from build123d import *

# Parameters (mm, degrees)
F1_DEPTH = 3.175
F2_R     = 1.984375
F3_DEPTH = 3.176


with BuildPart() as f1:
    # F0 (on Top) → F1 (new body)
    with BuildSketch(Plane.XY):
        with BuildLine():
            Line((75.480408, 88.9), (-75.480408, 88.9))
            Line((-75.480408, 88.9), (-75.480408, -88.9))
            Line((-75.480408, -88.9), (-100.880408, -88.9))
            Line((-100.880408, -88.9), (-100.880408, -101.6))
            ThreePointArc((-100.880408, -101.6), (0, -144.660291), (100.880408, -101.6))
            Line((100.880408, -101.6), (100.880408, -88.9))
            Line((100.880408, -88.9), (75.480408, -88.9))
            Line((75.480408, -88.9), (75.480408, 88.9))
        make_face()
    extrude(amount=F1_DEPTH)

    # F2 (on Top) → F3 (cut, through all)
    with BuildSketch(Plane.XY):
        with Locations((69.130408, -45.22089)):
            Circle(F2_R)
        with Locations((69.130408, -18.27911)):
            Circle(F2_R)
        with Locations((-69.130408, -45.22089)):
            Circle(F2_R)
        with Locations((-69.130408, -18.27911)):
            Circle(F2_R)
    extrude(amount=F3_DEPTH, mode=Mode.SUBTRACT)


solid = f1.part
Geometry check sheet. Reference: the model listing, model coordinates, mm. Round coordinates to 2 decimals unless told otherwise and drop trailing zeros. Order: outer loops, then holes, each group sorted by start corner. A loop starts at its lowest first (then second) coordinate and runs counter-clockwise, first axis right, second up. Notation, with made-up numbers: (12, -11) - (61, -11) arc R19 ccw to (61, 9) - close; hole circle Ø1 at (65, -25.5). An arc over 180 degrees is marked (long way). One line per question, with ' | ' between items. Start each with the question number.
(1) Sectioned sample at B-B on z = 1.1. Record the cut outline in (x, y), and give its area (3 significant figures).
(2) Depth check by flat-ended pin: pin 1 Ø2.5 at (x, y) = (69.13, -18.28) entering from +Z; pin 2 Ø1 at (y, z) = (-14.5, 1.5) entering from -X. Enter the tip coordinate at first touch or a pass-through.
(3) Sectioned sample at C-C on x = 32. Record the cut outline in (y, z) (3 decimals).
(4) Release check for a two-part mould opening along Y. For faces 1 (the cylindrical face through (-1.58, -144.65, 1.57)), 2 (the flat face through (-1, -26, 3.175)) record: released by +Y, released by -Y, zero draft, split by the parting line, or undercut.
(5) Thickness scan on L1, parallel to Y at x = 67.5, z = 1.35; L2, parallel to X at y = 52.5, z = 1.25; L3, parallel to Y at x = 2, z = 3. Record the ranges inside material, lowest first. Write a range as [from, to].
(6) Sectioned sample at A-A on y = 18. Record the cut outline in (x, z) (3 decimals).
Conclusion:
1) outline: (-100.88, -101.6) arc R139.7 ccw to (100.88, -101.6) - (100.88, -88.9) - (75.48, -88.9) - (75.48, 88.9) - (-75.48, 88.9) - (-75.48, -88.9) - (-100.88, -88.9) - close; hole circle Ø3.97 at (-69.13, -45.22); hole circle Ø3.97 at (-69.13, -18.28); hole circle Ø3.97 at (69.13, -45.22); hole circle Ø3.97 at (69.13, -18.28) | area: 35,400 mm2
2) pin 1: passes through | pin 2: stops at x = -75.48
3) outline: (-140.946, 0) - (88.9, 0) - (88.9, 3.175) - (-140.946, 3.175) - close
4) face 1: released by -Y | face 2: zero draft
5) L1: y = [-127.27, -46.35], [-44.09, -19.41], [-17.15, 88.9] | L2: x = [-75.48, 75.48] | L3: y = [-144.65, 88.9]
6) outline: (-75.48, 0) - (75.48, 0) - (75.48, 3.175) - (-75.48, 3.175) - close
